The model under review builds one solid part; all positions refer to its coordinate system, in mm. Coordinates: 2 decimals unless noted, no trailing zeros. Loops run counter-clockwise (first coordinate to the right, second up) from the corner with the lowest first, then second, coordinate; pieces in that order, holes last. Notation, with made-up numbers: M -10,42.25 L 44,42.25 A10 cw 44,52.25 Z; hole C -10.75,-19.5 d11. An arc over 180 degrees is marked long. Write item = value, one per line. Start each with the question number.
Q1. Clearance check with a flat-ended pin moving along its axis: pin 1 Ø9 at (x, y) = (0, 0) entering from +Z. State where the tip first meets the part, or that it passes through.
Q2. Mouldability with a two-part tool opening along X and no side actions: class faces 1 (the face through (-30, 5, 5)), 2 (the face through (0, -18.5, 5)), 3 (the face through (-0.867, -3.905, 5.07)) as released by +X, released by -X, zero draft, split by the parting line, or undercut.
Q3. We need section A-A on y = 0. Give the boundary of the cut face in (x, z).
Q4. Wall thickness on probe 1 along X at (y, z) = (-1, 8.75); probe 2 along Y at (x, z) = (-20, 7.5); probe 3 along X at (y, z) = (-0.5, 2.75): over which ranges is each line inside the solid? List them lowest first.
Q5. We need section D-D on x = -17. Give the boundary of the cut face in (y, z).
Q6. We need section B-B on x = 0. Give the boundary of the cut face in (y, z).
Q7. We need section C-C on z = 1.75. Give the boundary of the cut face in (x, y).
from build123d import *

# Parameters (mm, degrees)
ESQUISSE1_W             = 60
ESQUISSE1_H             = 50
BASE_EXTRUSION_DEPTH    = 10
CONG_1_R                = 3
ESQUISSE2_R             = 4
ENL_V_MAT_EXTRU_1_DEPTH = 10


with BuildPart() as part:
    # Esquisse1 → Base-Extrusion (new body)
    with BuildSketch(Plane.XY):
        with Locations((0, 6.5)):
            Rectangle(ESQUISSE1_W, ESQUISSE1_H)
    extrude(amount=BASE_EXTRUSION_DEPTH)

    # Congé1
    cong_1_edges = [part.edges().sort_by_distance(p)[0] for p in [
        (30, 31.5, 5),
        (-30, 31.5, 5),
    ]]
    fillet(cong_1_edges, radius=CONG_1_R)

    # Esquisse2 → Enlèv. mat.-Extru.1 (cut)
    with BuildSketch(Plane.XY.offset(10)):
        with Locations((-20, 0)):
            Circle(ESQUISSE2_R)
        Circle(ESQUISSE2_R)
        with Locations((20, 0)):
            Circle(ESQUISSE2_R)
    extrude(amount=-ENL_V_MAT_EXTRU_1_DEPTH, mode=Mode.SUBTRACT)


solid = part.part
Returned:
q1.pin_1 = 10
q2.face_1 = released by -X
q2.face_2 = zero draft
q2.face_3 = undercut
q3.outline = M -30,0 L -24,0 L -24,10 L -30,10 Z; M -16,0 L -4,0 L -4,10 L -16,10 Z; M 4,0 L 16,0 L 16,10 L 4,10 Z; M 24,0 L 30,0 L 30,10 L 24,10 Z
q4.probe_1 = -30 to -23.87, -16.13 to -3.87, 3.87 to 16.13, 23.87 to 30
q4.probe_2 = -18.5 to -4, 4 to 31.5
q4.probe_3 = -30 to -23.97, -16.03 to -3.97, 3.97 to 16.03, 23.97 to 30
q5.outline = M -18.5,0 L -2.65,0 L -2.65,10 L -18.5,10 Z; M 2.65,0 L 31.5,0 L 31.5,10 L 2.65,10 Z
q6.outline = M -18.5,0 L -4,0 L -4,10 L -18.5,10 Z; M 4,0 L 31.5,0 L 31.5,10 L 4,10 Z
q7.outline = M -30,-18.5 L 30,-18.5 L 30,28.5 A3 ccw 27,31.5 L -27,31.5 A3 ccw -30,28.5 Z; hole C -20,0 d8; hole C 0,0 d8; hole C 20,0 d8
